Print and shaded views of the part. All mm, measured from the part's lowest x, y and z. A direction names the side the tool comes from. Coordinates: 2 decimals unless noted, no trailing zeros. Loops run counter-clockwise (first coordinate to the right, second up) from the corner with the lowest first, then second, coordinate; pieces in that order, holes last.
1) Saw through at C-C, the plane y = 3.25. Write the cut outline in (x, z), and give its area (3 significant figures).
2) Saw through at D-D, the plane z = 45. Write the cut outline in (x, y), and give its area (3 significant figures).
3) Saw through at A-A, the plane x = 6. Write the cut outline in (y, z), and give its area (3 significant figures).
4) Pin check, flat tips, straight feed: pin 1 Ø1 at (x, y) = (4, 5) entering from -Z; pin 2 Ø4 at (x, y) = (1.5, 7.5) entering from +Z; pin 3 Ø5 at (x, z) = (6, 42.5) entering from +Y; pin 4 Ø1 at (x, z) = (10.5, 29.5) entering from -Y. Stop position of each tip, or through.
5) Which spindle directions (+Z, -Z, +X, -X, +Y, -Y) get a long thin tool onto all of the face, cutting with end or side? Do the marked faces 1, 2 and 3. Say none if no direction does.
6) Wall check: line 1 along Z through (x, y) = (8.25, 3); line 2 along Y through (x, z) = (6.5, 45) (1 decimal); line 3 along Y through (x, z) = (8.5, 57.5) (1 decimal). Give the ranges that are in metal, low to high.
7) Saw through at B-B, the plane z = 33. Write the cut outline in (x, y).
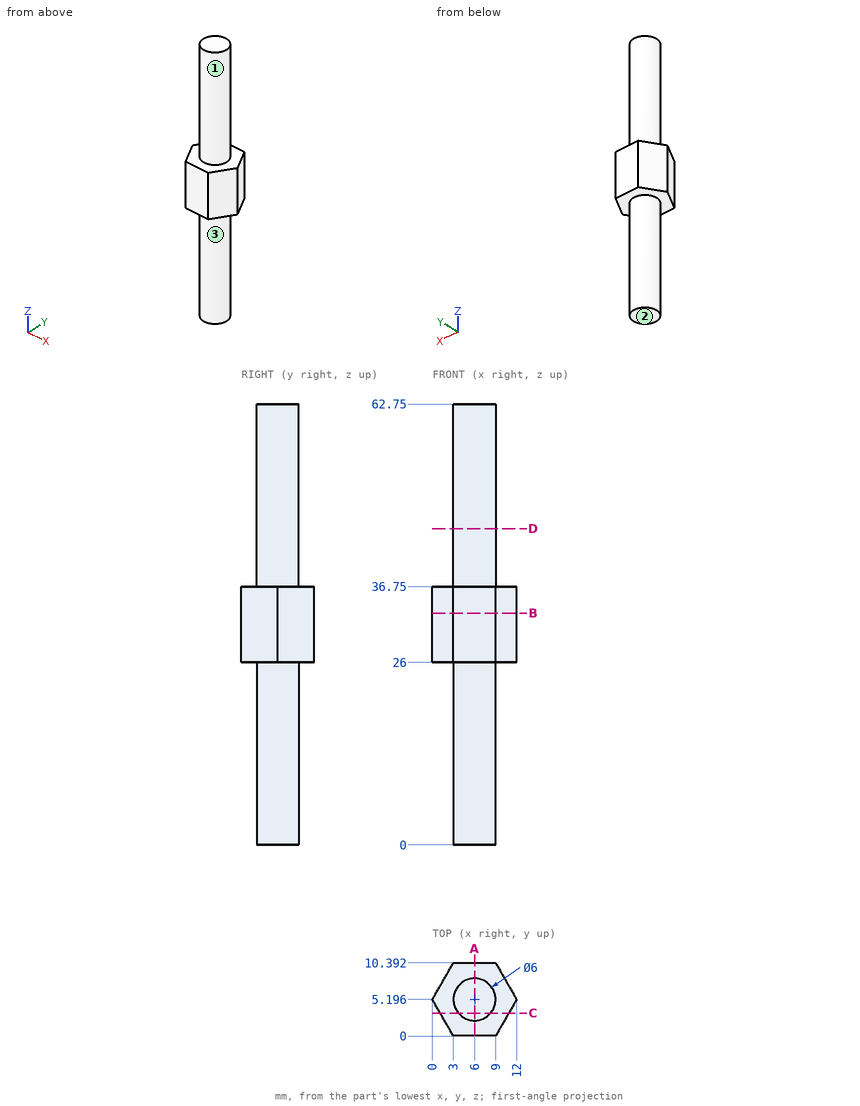
Data:
1. outline: (1.12, 26) - (3.72, 26) - (3.72, 0) - (8.28, 0) - (8.28, 26) - (10.88, 26) - (10.88, 36.75) - (8.28, 36.75) - (8.28, 62.75) - (3.72, 62.75) - (3.72, 36.75) - (1.12, 36.75) - close
1. area: 342 mm2
2. outline: circle Ø6 at (6, 5.2)
2. area: 28.3 mm2
3. outline: (0, 26) - (2.2, 26) - (2.2, 0) - (8.2, 0) - (8.2, 26) - (10.39, 26) - (10.39, 36.75) - (8.2, 36.75) - (8.2, 62.75) - (2.2, 62.75) - (2.2, 36.75) - (0, 36.75) - close
3. area: 424 mm2
4. pin 1: stops at z = 0
4. pin 2: stops at z = 36.75
4. pin 3: stops at y = 8.2
4. pin 4: stops at y = 1.73
5. face 1: +Z
5. face 2: -Z, +X, -X, +Y, -Y
5. face 3: -Z
6. line 1: z = 26 to 36.75
6. line 2: y = 2.2 to 8.2
6. line 3: y = 3.5 to 6.9
7. outline: (0, 5.2) - (3, 0) - (9, 0) - (12, 5.2) - (9, 10.39) - (3, 10.39) - close
